Input: dimensioned drawing with shaded views. Units: mm. Origin: part minimum x, y, z. Give positions to 0.01 mm unless a question says otherwise; leave off trailing zeros. Write each loop counter-clockwise with the first axis right and the second up, starting at its lowest first coordinate (ties: lowest second). Pieces come first, ordered by that corner, then holes. Notation, with made-up numbers: M -13,-16.5 L -3,-16.5 A19 ccw -3,-1.5 Z; hole C 80.5,5 d6. An arc over 180 degrees is marked long. Answer as a JSON object with one key per item and string values.
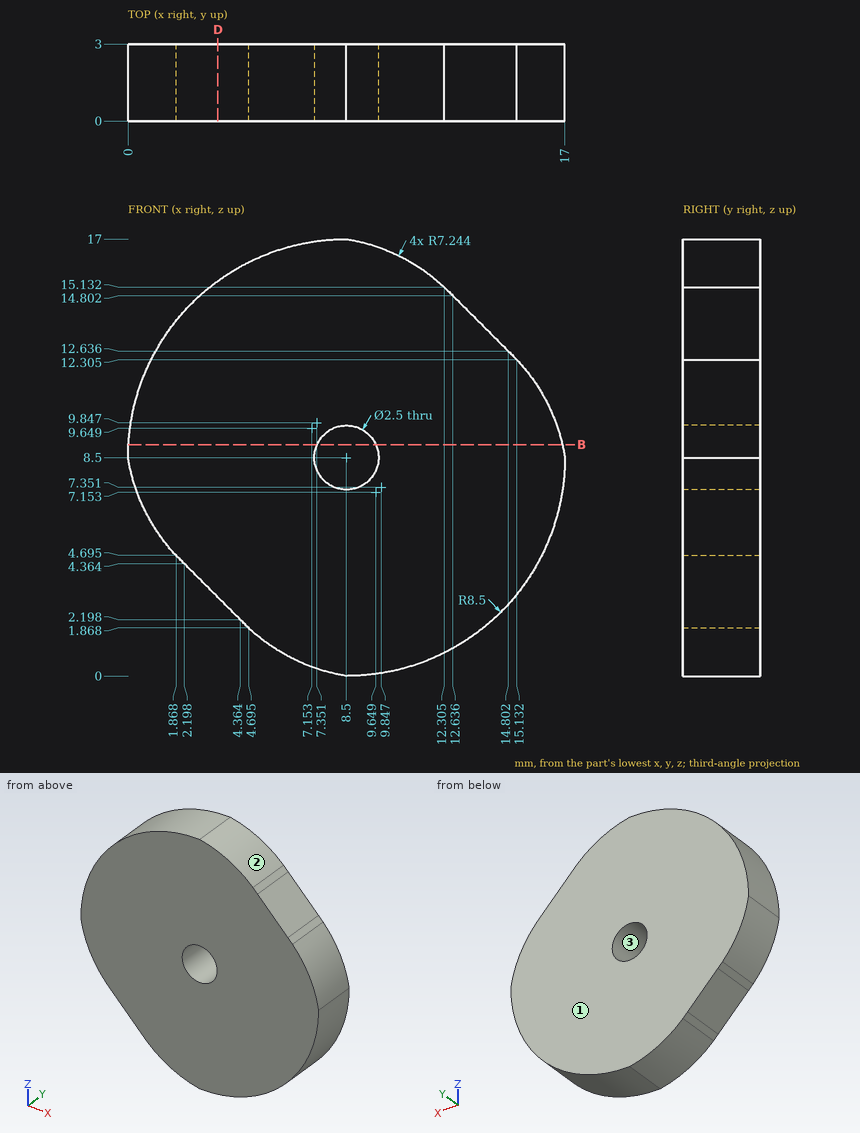
1) Pull-direction query (Z, two-part tool) for the marked faces 1, 2 and 3; classes: pulls with the +Z half, pulls with the -Z half, needs draft (parallel to the pull), parting line crosses it, or undercut.
Geometry check:
{"face 1": "needs draft", "face 2": "pulls with the +Z half", "face 3": "undercut"}
2) Cut plane D-D on x = 3.5. Return loops of the section in (y, z).
Geometry check:
{"outline": "M 0,3.06 L 3,3.06 L 3,15.37 L 0,15.37 Z"}
3) Cut plane B-B on z = 9. Return loops of the section in (x, y) (1 decimal).
Geometry check:
{"outline": "M 0,0 L 7.4,0 L 7.4,3 L 0,3 Z; M 9.6,0 L 16.9,0 L 16.9,3 L 9.6,3 Z"}
4) Line query: line 1 (Z direction, x = 8.5, y = 1.4); line 2 (Z direction, x = 9.25, y = 2.9) (1 decimal). Output: solid intervals per line, ascending. Write a range as from..to.
Geometry check:
{"line 1": "z = 0..7.25, 9.75..17", "line 2": "z = 0..7.5, 9.5..16.8"}
